from build123d import *

# Parameters (mm, degrees)
ESQUISSE4_W        = 1.2
ESQUISSE4_H        = 7.846267026
BOSS_EXTRU_1_DEPTH = 6.35


with BuildPart() as part:
    # Esquisse1 → Révolution1 (revolve)
    with BuildSketch(Plane.XY):
        with BuildLine():
            Line((3.96875, 0), (3.96875, 9.534696006))
            ThreePointArc((3.96875, 9.534696006), (5.270377511, 15.960075858), (8.970022713, 21.372318074))
            Line((8.970022713, 21.372318074), (39.238684771, 50.8))
            Line((39.238684771, 50.8), (38.1, 50.8))
            Line((38.1, 50.8), (8.176272713, 21.707669228))
            ThreePointArc((8.176272713, 21.707669228), (4.476627511, 16.295427012), (3.175, 9.87004716))
            Line((3.175, 9.87004716), (3.175, 0))
            Line((3.175, 0), (3.96875, 0))
        make_face()
    revolve(axis=Axis((0, 0, 0), (0, 1, 0)))

    # Esquisse4 → Boss.-Extru.1 (add)
    with BuildSketch(Plane.XZ):
        Rectangle(ESQUISSE4_W, ESQUISSE4_H)
    extrude(amount=-BOSS_EXTRU_1_DEPTH)


solid = part.part
Can you work these out from the model? Positions are in its coordinate system, mm. A direction names the side the tool comes from. Coordinates: 2 decimals unless noted, no trailing zeros. Write each loop counter-clockwise with the first axis right and the second up, starting at its lowest first coordinate (ties: lowest second). Pieces come first, ordered by that corner, then holes. Notation, with made-up numbers: (65.25, -31.5) -> (101.25, -31.5) arc R5 cw to (101.25, -24.5) -> close; hole circle Ø5 at (56, 76). An arc over 180 degrees is marked (long way). Answer as CSV lines item,"result".
1) If we section it at C-C on y = 17: Please give me the cut outline in (x, z).
Check result:
outline,"circle Ø11.51 at (0, 0); hole circle Ø9.59 at (0, 0)"
2) If we mould it in two halves opening along X, with no side actions, what happens to faces 4 (the conical face through (10.36, 23.21, -3.26)), 5 (the flat face through (-21, 50.8, -32)), 6 (the conical face through (9.185, 23.12, -2.892)), 7 (the cylindrical face through (1.5, 4.9, 2.8))? For each: +X half, -X half, draft (parallel to the pull), parting line (faces both ways), or undercut.
Check result:
face 4,"parting line"
face 5,"draft"
face 6,"undercut"
face 7,"undercut"
3) If we section it at A-A on z = 0: Please give me the cut outline in (x, y) (3 decimals), then the cut area to 3 significant figures.
Check result:
outline,"(-39.239, 50.8) -> (-8.97, 21.372) arc R16.51 cw to (-3.969, 9.535) -> (-3.969, 0) -> (-3.175, 0) -> (-3.175, 9.87) arc R16.51 ccw to (-8.176, 21.708) -> (-38.1, 50.8) -> close; (-0.6, 0) -> (0.6, 0) -> (0.6, 6.35) -> (-0.6, 6.35) -> close; (3.175, 0) -> (3.969, 0) -> (3.969, 9.535) arc R16.51 cw to (8.97, 21.372) -> (39.239, 50.8) -> (38.1, 50.8) -> (8.176, 21.708) arc R16.51 ccw to (3.175, 9.87) -> close"
area,"112 mm²"
4) Will these pins go through, and if not, where does the flat tip stop? P1, Ø8, axis at y = 41, z = 15.5, coming from the +X side; P2, Ø12, axis at x = 22, z = -5, coming from the +Y side; P3, Ø1.9, axis at y = 4.5, z = -0.5, coming from the -X side; P4, Ø4, axis at x = -2.5, z = 1.5, coming from the -Y side.
Check result:
P1,"x = 29.85"
P2,"y = 41.53"
P3,"x = -3.97"
P4,"y = 0"
5) If I drill on line 1 (X direction, y = 2.5, z = 0) (3 decimals); line 2 (Z direction, x = 0, y = 7) (3 decimals), over which ranges is the centre line in solid material (lowest first)? Write a range as from..to.
Check result:
line 1,"-3.969..-3.175, -0.6..0.6, 3.175..3.969"
line 2,"-3.969..-3.175, 3.175..3.969"
6) If we section it at B-B on y = 30.5: Please give me the cut outline in (x, z), then the cut area to 3 significant figures.
Check result:
outline,"circle Ø36.72 at (0, 0); hole circle Ø34.44 at (0, 0)"
area,"127 mm²"
7) On a 3-axis mill with a long thin cutter (end or side, diameter ignored), from which of +Z, -Z, +X, -X, +Y, -Y can I reach the whole of each face in a straight line? I mean faces 1 (the flat face through (-0.6, 3, 0)), 2 (the cylindrical face through (-0.86, 4.834, 3.874)), 3 (the flat face through (0, 0, 0)). Say none if no direction works.
Check result:
face 1,"+Y, -Y"
face 2,"-Y"
face 3,"+Z, -Z, +X, -X, -Y"
